The model under review builds one solid part; all positions refer to its coordinate system, in mm. Face numbers are marked on the shaded views. Give positions to 0.01 mm unless a question says otherwise; leave off trailing zeros. Order: outer loops, then holes, each group sorted by start corner. A loop starts at its lowest first (then second) coordinate and runs counter-clockwise, first axis right, second up. Notation, with made-up numbers: (64, -12.75) - (106, -12.75) arc R18 cw to (106, 8.25) - close; hole circle Ø6 at (78.5, 33). An arc over 180 degrees is marked (long way). Put each result on its own line as item: value.
```python
from build123d import *

# Parameters (mm, degrees)
BOSS_EXTRUDE1_DEPTH = 3
SKETCH2_W           = 4
SKETCH2_H           = 15.5
BOSS_EXTRUDE2_DEPTH = 1
CUT_EXTRUDE1_DEPTH  = 0.25


with BuildPart() as part:
    # Sketch1 → Boss-Extrude1 (new body)
    with BuildSketch(Plane(origin=(0, 0, 0), x_dir=(1, 0, 0), z_dir=(0, 1, 0))):
        Polygon((-1, -7.25), (1, -7.25), (1, 7.25), (2, 7.25), (2, -7.25), (2, -8.25), (1, -8.25), (-2, -8.25), (-2, 7.25), (-1, 7.25), align=None)
    extrude(amount=BOSS_EXTRUDE1_DEPTH)

    # Sketch2 → Boss-Extrude2 (add)
    with BuildSketch(Plane(origin=(0, 3, 0), x_dir=(1, 0, 0), z_dir=(0, 1, 0))):
        with Locations((0, -0.5)):
            Rectangle(SKETCH2_W, SKETCH2_H)
    extrude(amount=BOSS_EXTRUDE2_DEPTH)

    # Sketch3 → Cut-Extrude1 (cut)
    with BuildSketch(Plane.XZ):
        Polygon((-1, 7.25), (1, 7.25), (1, -7.25), (1.5, -7.25), (1.5, 7.717200742), (-1.5, 7.717200742), (-1.5, -7.25), (-1, -7.25), align=None)
    extrude(amount=-CUT_EXTRUDE1_DEPTH, mode=Mode.SUBTRACT)


solid = part.part
```
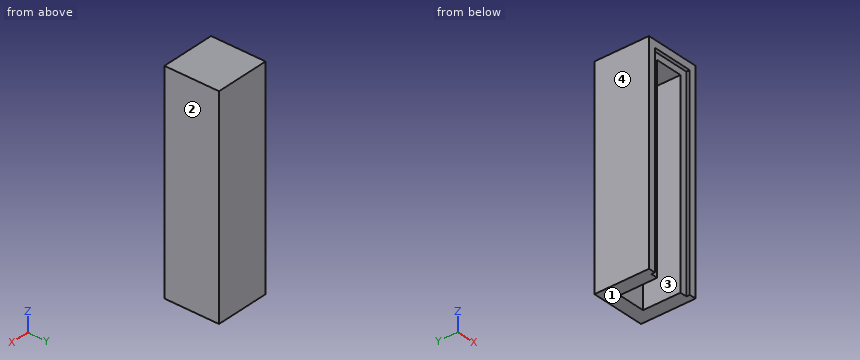
(1) The part is to be moulded in two halves that separate along X. For the marked faces 1, 2, 3 and 4, say which applies: pulls with the +X half, pulls with the -X half, needs draft (parallel to the pull), parting line crosses it, or undercut.
The answers:
face 1: needs draft
face 2: pulls with the +X half
face 3: undercut
face 4: pulls with the -X half
(2) Take a section at D-D, the plane x = -0.35. Write out the cut boundary in (y, z), then the cut area to 3 significant figures.
The answers:
outline: (0, 7.72) - (0.25, 7.72) - (0.25, 7.25) - (3, 7.25) - (3, -7.25) - (4, -7.25) - (4, 8.25) - (0, 8.25) - close
area: 18.4 mm^2
(3) Take a section at B-B, the plane y = 1.95. Write out the cut boundary in (x, z), then the cut area to 3 significant figures.
The answers:
outline: (-2, -7.25) - (-1, -7.25) - (-1, 7.25) - (1, 7.25) - (1, -7.25) - (2, -7.25) - (2, 8.25) - (-2, 8.25) - close
area: 33.0 mm^2
(4) Take a section at A-A, the plane z = -5. Write out the cut boundary in (x, y), then the cut area to 3 significant figures.
The answers:
outline: (-2, 0) - (-1.5, 0) - (-1.5, 0.25) - (-1, 0.25) - (-1, 3) - (1, 3) - (1, 0.25) - (1.5, 0.25) - (1.5, 0) - (2, 0) - (2, 4) - (-2, 4) - close
area: 9.75 mm^2
(5) Take a section at C-C, the plane x = -1.35. Write out the cut boundary in (y, z), then the cut area to 3 significant figures.
The answers:
outline: (0, 7.72) - (0.25, 7.72) - (0.25, -7.25) - (4, -7.25) - (4, 8.25) - (0, 8.25) - close
area: 58.3 mm^2
(6) Wall thickness on L1, parallel to X at y = 1.2, z = -2.25; L2, parallel to Y at x = 1.4, z = 7.25; L3, parallel to Y at x = -0.4, z = 3.75: over which ranges is each line inside the solid? List them lowest first.
The answers:
L1: -2 to -1, 1 to 2
L2: 0.25 to 4
L3: 3 to 4
(7) Clearance check with flat-ended pins moving along their axes: pin 1 Ø0.6 at (x, z) = (0, 2) entering from -Y; pin 2 Ø0.6 at (x, y) = (0, 2) entering from -Z. State where each tip first meets the part, or that it passes through.
The answers:
pin 1: y = 3
pin 2: z = 7.25
